Model file for the job. Use its own axes, mm. Round coordinates to 2 decimals unless told otherwise and drop trailing zeros. Loops run counter-clockwise (first coordinate to the right, second up) from the corner with the lowest first, then second, coordinate; pieces in that order, holes last. Notation, with made-up numbers: (60, -26.75) -> (91, -26.75) arc R24 cw to (91, -2.75) -> close; hole circle Ø3 at (39, 30). An arc over 180 degrees is marked (long way). Use a Markdown table: item, result. Add a question column.
```python
from build123d import *

# Parameters (mm, degrees)
SKETCH1_W           = 129.54
SKETCH1_H           = 129.54
SKETCH1_R           = 2.667
SKETCH1_W_2         = 114.3
SKETCH1_H_2         = 114.3
SKETCH1_H_3         = 4.852699468
SKETCH1_W_3         = 4.852699468
BOSS_EXTRUDE1_DEPTH = 2.54


with BuildPart() as part:
    # Sketch1 → Boss-Extrude1 (new body)
    # profile 1 of 3: a face of its own
    with BuildSketch(Plane(origin=(0, 0, 0), x_dir=(1, 0, 0), z_dir=(0, 1, 0))):
        Rectangle(SKETCH1_W, SKETCH1_H)
        with Locations(Location((-60.198, -60.198, 0), (0, 0, 270))):
            Circle(SKETCH1_R, mode=Mode.SUBTRACT)
        with Locations(Location((60.198, -60.198, 0), (0, 0, 270))):
            Circle(SKETCH1_R, mode=Mode.SUBTRACT)
        with Locations(Location((-60.198, 60.198, 0), (0, 0, 270))):
            Circle(SKETCH1_R, mode=Mode.SUBTRACT)
        with Locations(Location((60.198, 60.198, 0), (0, 0, 270))):
            Circle(SKETCH1_R, mode=Mode.SUBTRACT)
        Rectangle(SKETCH1_W_2, SKETCH1_H_2, mode=Mode.SUBTRACT)
    # profile 2 of 3: a face of its own
    with BuildSketch(Plane(origin=(0, 0, 0), x_dir=(1, 0, 0), z_dir=(0, 1, 0))):
        Rectangle(SKETCH1_W, SKETCH1_H_3)
    # profile 3 of 3: a face of its own
    with BuildSketch(Plane(origin=(0, 0, 0), x_dir=(1, 0, 0), z_dir=(0, 1, 0))):
        Rectangle(SKETCH1_W_3, SKETCH1_H)
    extrude(amount=BOSS_EXTRUDE1_DEPTH)


solid = part.part
```
1) Pin check, flat tips, straight feed: pin 1 Ø5 at (x, z) = (60.198, 60.198) entering from +Y; pin 2 Ø7 at (x, z) = (-60.198, 60.198) entering from +Y. Stop position of each tip, or through.
2) Pull direction X, two halves, no side cores. Call faces 1 (the face through (-61.821, 1.252, -62.314)), 2 (the face through (-15, 0, -1)): +X half, -X half, draft (parallel to the pull), parting line (faces both ways), or undercut.
3) Wall check: probe 1 along X at (y, z) = (2.45, 5.5). Give the ranges that are in metal, low to high. Write a range as from..to.
4) Cut at C-C on y = 0.75. Count the separate pieces of the cut face and the enclosed holes in it, and give its area (3 significant figures).
5) Cut at A-A on z = 38. Write the cut outline in (x, y), and give its area (3 significant figures).
6) Cut at B-B on x = 42. Write the cut outline in (y, z).
Established:
| question | item | result |
|---|---|---|
| 1 | pin 1 | passes through |
| 1 | pin 2 | stops at y = 2.54 |
| 2 | face 1 | undercut |
| 2 | face 2 | draft |
| 3 | probe 1 | x = -64.77..-57.15, -2.43..2.43, 57.15..64.77 |
| 4 | separate pieces | 1 |
| 4 | enclosed holes | 8 |
| 4 | area | 4,710 mm^2 |
| 5 | outline | (-64.77, 0) -> (-57.15, 0) -> (-57.15, 2.54) -> (-64.77, 2.54) -> close; (-2.43, 0) -> (2.43, 0) -> (2.43, 2.54) -> (-2.43, 2.54) -> close; (57.15, 0) -> (64.77, 0) -> (64.77, 2.54) -> (57.15, 2.54) -> close |
| 5 | area | 51.0 mm^2 |
| 6 | outline | (0, -64.77) -> (2.54, -64.77) -> (2.54, -57.15) -> (0, -57.15) -> close; (0, -2.43) -> (2.54, -2.43) -> (2.54, 2.43) -> (0, 2.43) -> close; (0, 57.15) -> (2.54, 57.15) -> (2.54, 64.77) -> (0, 64.77) -> close |
